Autodesk Inventor part; units mm, degrees
ref_plane "YZ Plane" through (0, 0, 0) normal (1, 0, 0) x (0, 1, 0)
ref_plane "XZ Plane" through (0, 0, 0) normal (0, 1, 0) x (-1, 0, 0)
ref_plane "XY Plane" through (0, 0, 0) normal (0, 0, 1) x (1, 0, 0)
sketch "Sketch1" plane through (0, 0, 0) normal (0, 0, 1) x (1, 0, 0)
  line L0 (-166.5857, -260.2376) -> (112.8143, -260.2376)
  line L1 (112.8143, -260.2376) -> (112.8143, 136.6374)
  line L2 (112.8143, 136.6374) -> (-166.5857, 136.6374)
  line L3 (-166.5857, 136.6374) -> (-166.5857, -260.2376)
  point P0 (0, 0)
  dimension "d0" = 396.875
  dimension "d3" = 279.4
extrude "Board" add sketch "Sketch1" along normal blind 6.35
sketch "Sketch2" plane through (0, 0, 6.35) normal (0, 0, 1) x (1, 0, 0)
  circle A0 centre (-90.3857, -61.8001) radius 19.05
  line L0 (-166.5857, -260.2376) -> (112.8143, -260.2376)
  line L1 (-166.5857, 136.6374) -> (-166.5857, -260.2376)
  line L2 (112.8143, -260.2376) -> (112.8143, 136.6374)
  line L3 (112.8143, -112.6001) -> (87.4143, -112.6001)
  line L4 (62.0143, -87.2001) -> (62.0143, -36.4001)
  line L5 (87.4143, -11.0001) -> (112.8143, -11.0001)
  line L6 (112.8143, -11.0001) -> (112.8143, -112.6001)
  arc A1 (62.0143, -87.2001) -> (87.4143, -112.6001) centre (87.4143, -87.2001) ccw
  arc A2 (87.4143, -11.0001) -> (62.0143, -36.4001) centre (87.4143, -36.4001) ccw
  line L7 (112.8143, 136.6374) -> (-166.5857, 136.6374)
  point P0 (0, 0)
  point P1 (62.0143, -11.0001)
  dimension "d4" = 38.1
  dimension "d5" = 198.4375
  dimension "d6" = 76.2
  dimension "d9" = 50.8
  dimension "d10" = 25.4
  dimension "d11" = 101.6
  dimension "d12" = 25.4
  dimension "d13" = 147.6375
extrude "Cutout Holes" cut sketch "Sketch2" against normal blind 6.35 contours A0 | L3 A1 L4 A2 L5 L2
equation "\"d5\" = 0.5 * d0"
equation "\"d13\" = -0.5 * d11 + 0.5 * d0"
properties part number "Back Panel Bottom"
CAD build for the part. Positions are in the model's coordinates, mm. A direction names the side the tool comes from. Coordinates: 2 decimals unless noted, no trailing zeros. Order: outer loops, then holes, each group sorted by start corner. A loop starts at its lowest first (then second) coordinate and runs counter-clockwise, first axis right, second up. Notation, with made-up numbers: (52.5, -34) -> (83.5, -34) arc R10 ccw to (83.5, -27) -> close; hole circle Ø8 at (-32.5, -29.75). An arc over 180 degrees is marked (long way). Use one line per item in the form item = value. Start each with the question number.
1) Band-saw the part on A-A on x = -85.5. Give the cut face in (y, z), then the cut area to 3 significant figures.
2) Band-saw the part on C-C on y = -97.5. Give the cut face in (x, z).
3) Drill centre lines: L1, parallel to X at y = -73.5, z = 4.75; L2, parallel to Y at x = 78.5, z = 2; L3, parallel to Y at x = -94, z = 3.5. Where is each one in solid material? Low to high. Write a range as [from, to].
4) Pull direction Y, two halves, no side cores. Call faces 3 (the flat face through (-29, -59, 0)), 4 (the cylindrical face through (69.257, -104.962, 3.219)): +Y half, -Y half, draft (parallel to the pull), parting line (faces both ways), or undercut.
5) Tool access for faces 1 (the flat face through (-29, -59, 6.35)), 2 (the cylindrical face through (69.652, -18.243, 3.219)): list every direction of +Z, -Z, +X, -X, +Y, -Y with a clear straight run to the whole face (end or side of a thin tool).
6) Band-saw the part on B-B on z = 2. Give the cut face in (x, y).
Entries:
q1.outline = (-260.24, 0) -> (-80.21, 0) -> (-80.21, 6.35) -> (-260.24, 6.35) -> close; (-43.39, 0) -> (136.64, 0) -> (136.64, 6.35) -> (-43.39, 6.35) -> close
q1.area = 2,290 mm2
q2.outline = (-166.59, 0) -> (64.2, 0) -> (64.2, 6.35) -> (-166.59, 6.35) -> close
q3.L1 = [-166.59, -105.42], [-75.35, 62.01]
q3.L2 = [-260.24, -110.98], [-12.62, 136.64]
q3.L3 = [-260.24, -80.5], [-43.1, 136.64]
q4.face_3 = draft
q4.face_4 = undercut
q5.face_1 = +Z, +X, -X, +Y, -Y
q5.face_2 = +Z, -Z, +X
q6.outline = (-166.59, -260.24) -> (112.81, -260.24) -> (112.81, -112.6) -> (87.41, -112.6) arc R25.4 cw to (62.01, -87.2) -> (62.01, -36.4) arc R25.4 cw to (87.41, -11) -> (112.81, -11) -> (112.81, 136.64) -> (-166.59, 136.64) -> close; hole circle Ø38.1 at (-90.39, -61.8)
